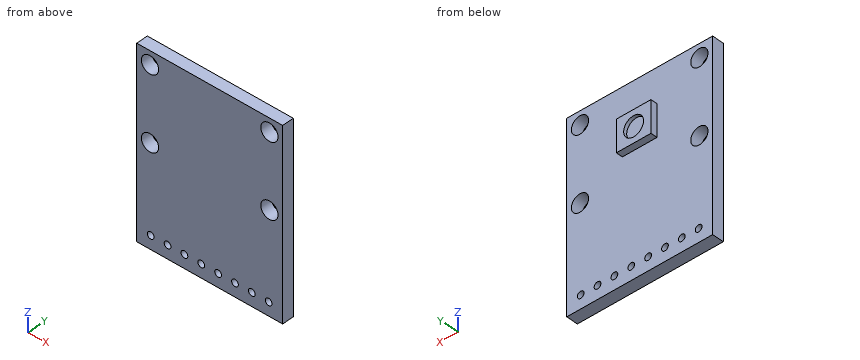
```python
from build123d import *

# Parameters (mm, degrees)
SKETCH1_W           = 22
SKETCH1_H           = 28
SKETCH1_R           = 1.3
SKETCH1_R_2         = 0.508
BOSS_EXTRUDE1_DEPTH = 1.75
SKETCH2_W           = 5.22
SKETCH2_H           = 4.75
BOSS_EXTRUDE2_DEPTH = 1
SKETCH3_R           = 1.5
CUT_EXTRUDE1_DEPTH  = 0.5


with BuildPart() as part:
    # Sketch1 → Boss-Extrude1 (new body)
    with BuildSketch(Plane(origin=(0, 0, 0), x_dir=(1, 0, 0), z_dir=(0, 1, 0))):
        with Locations((0, 6.5)):
            Rectangle(SKETCH1_W, SKETCH1_H)
        with Locations(Location((-9, 5.5, 0), (0, 0, 270))):
            Circle(SKETCH1_R, mode=Mode.SUBTRACT)
        with Locations(Location((9, 5.5, 0), (0, 0, 270))):
            Circle(SKETCH1_R, mode=Mode.SUBTRACT)
        with Locations(Location((9, -5.5, 0), (0, 0, 270))):
            Circle(SKETCH1_R, mode=Mode.SUBTRACT)
        with Locations(Location((-9, -5.5, 0), (0, 0, 270))):
            Circle(SKETCH1_R, mode=Mode.SUBTRACT)
        with Locations(Location((-8.89, 18.5, 0), (0, 0, 270))):
            Circle(SKETCH1_R_2, mode=Mode.SUBTRACT)
        with Locations(Location((-6.35, 18.5, 0), (0, 0, 270))):
            Circle(SKETCH1_R_2, mode=Mode.SUBTRACT)
        with Locations(Location((-3.81, 18.5, 0), (0, 0, 270))):
            Circle(SKETCH1_R_2, mode=Mode.SUBTRACT)
        with Locations(Location((-1.27, 18.5, 0), (0, 0, 270))):
            Circle(SKETCH1_R_2, mode=Mode.SUBTRACT)
        with Locations(Location((1.27, 18.5, 0), (0, 0, 270))):
            Circle(SKETCH1_R_2, mode=Mode.SUBTRACT)
        with Locations(Location((3.81, 18.5, 0), (0, 0, 270))):
            Circle(SKETCH1_R_2, mode=Mode.SUBTRACT)
        with Locations(Location((6.35, 18.5, 0), (0, 0, 270))):
            Circle(SKETCH1_R_2, mode=Mode.SUBTRACT)
        with Locations(Location((8.89, 18.5, 0), (0, 0, 270))):
            Circle(SKETCH1_R_2, mode=Mode.SUBTRACT)
    extrude(amount=BOSS_EXTRUDE1_DEPTH)

    # Sketch2 → Boss-Extrude2 (add)
    with BuildSketch(Plane(origin=(0, 1.75, 0), x_dir=(1, 0, 0), z_dir=(0, 1, 0))):
        Rectangle(SKETCH2_W, SKETCH2_H)
    extrude(amount=BOSS_EXTRUDE2_DEPTH)

    # Sketch3 → Cut-Extrude1 (cut)
    with BuildSketch(Plane(origin=(0, 2.75, 0), x_dir=(1, 0, 0), z_dir=(0, 1, 0))):
        with Locations(Location((0, 0, 0), (0, 0, 270))):
            Circle(SKETCH3_R)
    extrude(amount=-CUT_EXTRUDE1_DEPTH, mode=Mode.SUBTRACT)


solid = part.part
```
Check sheet for the modelled part. Datum: model origin and axes. Units: mm. Coordinates: 2 decimals unless noted, no trailing zeros. Loops run counter-clockwise (first coordinate to the right, second up) from the corner with the lowest first, then second, coordinate; pieces in that order, holes last. Notation, with made-up numbers: M -39.5,37.25 L -26.5,37.25 A23 ccw -26.5,58.25 Z; hole C 36.5,-35.5 d11. An arc over 180 degrees is marked long. Answer as a JSON object with one key per item and string values.
1. Depth check by flat-ended pin: P1, Ø1.3, axis at x = -6.35, z = -18.5, coming from the +Y side; P2, Ø1.6, axis at x = 9, z = -5.5, coming from the +Y side; P3, Ø1.1, axis at x = 1, y = 2.5, coming from the +Z side (3 decimals); P4, Ø0.5, axis at y = 2.5, z = 1, coming from the +X side. Enter the tip coordinate at first touch or a pass-through.
Outcome:
{"P1": "y = 1.75", "P2": "through", "P3": "z = 2.375", "P4": "x = 2.61"}
2. Sectioned sample at D-D on z = -12. Record the cut outline in (x, y).
Outcome:
{"outline": "M -11,0 L 11,0 L 11,1.75 L -11,1.75 Z"}
3. Sectioned sample at A-A on x = 6.35. Record the cut outline in (y, z), and give its area (3 significant figures).
Outcome:
{"outline": "M 0,-20.5 L 1.75,-20.5 L 1.75,-19.01 L 0,-19.01 Z; M 0,-17.99 L 1.75,-17.99 L 1.75,7.5 L 0,7.5 Z", "area": "47.2 mm²"}
4. Sectioned sample at C-C on z = -18.5. Count the separate pieces of the cut face and the enclosed holes in it, and give its area (3 significant figures).
Outcome:
{"separate pieces": "9", "enclosed holes": "0", "area": "24.3 mm²"}
5. Sectioned sample at B-B on z = 0. Record the cut outline in (x, y), and give its area (3 significant figures).
Outcome:
{"outline": "M -11,0 L 11,0 L 11,1.75 L 2.61,1.75 L 2.61,2.75 L 1.5,2.75 L 1.5,2.25 L -1.5,2.25 L -1.5,2.75 L -2.61,2.75 L -2.61,1.75 L -11,1.75 Z", "area": "42.2 mm²"}
6. Scan lines: L1, parallel to X at y = 1.05, z = 5.5; L2, parallel to X at y = 2.45, z = 0; L3, parallel to Z at x = 8, y = 0.8. Record each from-to range of solid material in increasing order. Write a range as from..to.
Outcome:
{"L1": "-11..-10.3, -7.7..7.7, 10.3..11", "L2": "-2.61..-1.5, 1.5..2.61", "L3": "-20.5..-6.33, -4.67..4.67, 6.33..7.5"}
